from build123d import *

# Parameters (mm, degrees)
F1_DEPTH = 4
F2_R     = 3
F3_DEPTH = 16


with BuildPart() as f1:
    # F0 (on Top) → F1 (new body)
    with BuildSketch(Plane.XY):
        Polygon((-2.886751, -5), (2.886751, -5), (5.773503, 0), (2.886751, 5), (-2.886751, 5), (-5.773503, 0), align=None)
    extrude(amount=F1_DEPTH)

    # F2 (on face) → F3 (join)
    with BuildSketch(Plane(origin=(0, 0, 0), x_dir=(1, 0, 0), z_dir=(0, 0, -1))):
        Circle(F2_R)
    extrude(amount=F3_DEPTH)

    # F4 (on Right) → F5 (revolve, cut)
    with BuildSketch(Plane.YZ):
        Polygon((9, 4), (5, 4), (9, 0), align=None)
    revolve(axis=Axis((0, 0, -1.209494), (0, 0, -1)), mode=Mode.SUBTRACT)


solid = f1.part
The model under review builds one solid part; all positions refer to its coordinate system, in mm. A direction names the side the tool comes from. Coordinates: 2 decimals unless noted, no trailing zeros. Loops run counter-clockwise (first coordinate to the right, second up) from the corner with the lowest first, then second, coordinate; pieces in that order, holes last. Notation, with made-up numbers: M 56,-17.5 L 71,-17.5 A23 ccw 71,6.5 Z; hole C 39.25,17.25 d1. An arc over 180 degrees is marked long. Put each result on its own line as item: value. Start each with the question number.
Q1. For faces 1 (the flat face through (0, -5, 2)), 2 (the cylindrical face through (-3, 0, -8)), list the 3-axis set-ups (+Z, -Z, +X, -X, +Y, -Y) from which the entire face can be reached by the end or side of a thin tool; tool diameter is ignored.
Q2. Add section A-A (z = 2). Write out the cut boundary in (x, y), and give its area (3 significant figures).
Q3. Clearance check with flat-ended pins moving along their axes: pin 1 (5 mm diameter, centred on y = -2.5, z = -11, fed in from +X); pin 2 (3 mm diameter, centred on x = -1, z = -5, fed in from -Y). State where each tip first meets the part, or that it passes through.
Q4. Wall thickness on line 1 (Z direction, x = 4, y = -1.25); line 2 (X direction, y = 2.5, z = -7.75); line 3 (X direction, y = 0.5, z = -3.25): over which ranges is each line inside the solid? List them lowest first.
Q5. Add section B-B (z = -15). Write out the cut boundary in (x, y).
Answers:
1. face 1: +Z, -Z, +X, -X, -Y
1. face 2: -Z
2. outline: M -5.77,0 L -2.89,-5 L 2.89,-5 L 5.77,0 L 2.89,5 L -2.89,5 Z
2. area: 86.6 mm^2
3. pin 1: stops at x = 3
3. pin 2: stops at y = -3
4. line 1: z = 0 to 4
4. line 2: x = -1.66 to 1.66
4. line 3: x = -2.96 to 2.96
5. outline: C 0,0 d6
